Geometry: final body of the model. Coordinates: model frame, mm. Round coordinates to 2 decimals unless told otherwise and drop trailing zeros. Write each loop counter-clockwise with the first axis right and the second up, starting at its lowest first coordinate (ties: lowest second). Pieces come first, ordered by that corner, then holes. Notation, with made-up numbers: M 74,59 L 116,59 A25 ccw 116,75 Z; hole C 51,64 d10. An arc over 180 degrees is marked long. Answer as CSV lines item,"result". Start each with the question number.
Q1. Section query D-D on z = 0.75. Give the number of separate pieces and of enclosed holes in the cut face, and give its area (3 significant figures).
Q2. Section query C-C on x = 0. Output: boundary loops of the cut face in (y, z), and give its area (3 significant figures).
Q3. First-contact query: pin 1 (1 mm diameter, centred on x = -10, y = 5, fed in from -Z); pin 2 (0.8 mm diameter, centred on x = 8, z = 1, fed in from +Y); pin 3 (8 mm diameter, centred on x = 0, y = 9.144, fed in from -Z); pin 4 (0.5 mm diameter, centred on y = -3, z = 0.5, fed in from -X). Flat tips, straight axial feed; report the tip coordinate or a pass-through.
Q4. Ray query, probe 1 along Y at (x, z) = (-9, 1.45); probe 2 along X at (y, z) = (8, 1.55) (3 decimals); probe 3 along X at (y, z) = (7.25, 1.5) (3 decimals). Return the intervals inside material, ascending.
Q5. Section query B-B on y = 2.75. Output: boundary loops of the cut face in (x, z) (1 decimal), and give its area (3 significant figures).
Q6. Section query A-A on x = -5.08. Output: boundary loops of the cut face in (y, z), and give its area (3 significant figures).
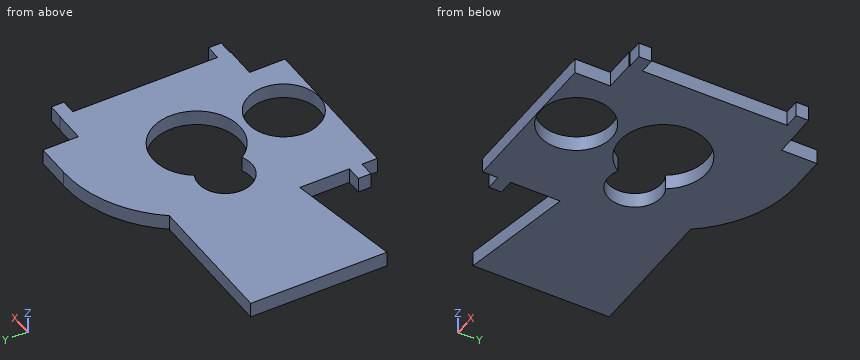
```python
from build123d import *

# Parameters (mm, degrees)
SKETCH1_R           = 3.7592
SKETCH1_W           = 1.5875
SKETCH1_H           = 1.3208
BOSS_EXTRUDE1_DEPTH = 1.5875
CUT_EXTRUDE1_REACH  = 32.926


with BuildPart() as part:
    # Sketch1 → Boss-Extrude1 (new body)
    # profile 1 of 6: a face of its own
    with BuildSketch(Plane.XY):
        with BuildLine():
            Line((2.54, 21.59), (9.525, 21.59))
            Line((9.525, 21.59), (9.525, -3.81))
            Line((9.525, -3.81), (-10.16, -3.81))
            Line((-10.16, -3.81), (-10.16, 8.89))
            ThreePointArc((-10.16, 8.89), (-6.440256121, 17.870256121), (2.54, 21.59))
        make_face()
        Circle(SKETCH1_R, mode=Mode.SUBTRACT)
        with BuildLine():
            ThreePointArc((-3.82905, 11.642311449), (-7.874, 9.144), (-3.82905, 6.645688551))
            ThreePointArc((-3.82905, 6.645688551), (4.572, 9.144), (-3.82905, 11.642311449))
        make_face(mode=Mode.SUBTRACT)
    # profile 2 of 6: a face of its own
    with BuildSketch(Plane.XY):
        with Locations((-10.95375, -1.5494)):
            Rectangle(SKETCH1_W, SKETCH1_H)
    # profile 3 of 6: a face of its own
    with BuildSketch(Plane.XY):
        with Locations((10.31875, 17.1704)):
            Rectangle(SKETCH1_W, SKETCH1_H)
    # profile 4 of 6: a face of its own
    with BuildSketch(Plane.XY):
        with Locations((10.31875, 0.6604)):
            Rectangle(SKETCH1_W, SKETCH1_H)
    # profile 5 of 6: a face of its own
    with BuildSketch(Plane.XY):
        with BuildLine():
            ThreePointArc((-10.16, 8.89), (-9.508277885, 12.906092628), (-7.62, 16.51))
            Line((-7.62, 16.51), (-22.084921519, 16.51))
            Line((-22.084921519, 16.51), (-22.084921519, 2.212007412))
            Line((-22.084921519, 2.212007412), (-10.16, 4.318))
            Line((-10.16, 4.318), (-10.16, 8.89))
        make_face()
    # profile 6 of 6: a face of its own
    with BuildSketch(Plane.XY):
        with BuildLine():
            ThreePointArc((-10.16, 8.89), (-9.508277885, 12.906092628), (-7.62, 16.51))
            Line((-7.62, 16.51), (-22.084921519, 16.51))
            Line((-22.084921519, 16.51), (-22.084921519, 2.212007412))
            Line((-22.084921519, 2.212007412), (-10.16, 4.318))
            Line((-10.16, 4.318), (-10.16, 8.89))
        make_face()
    extrude(amount=BOSS_EXTRUDE1_DEPTH)

    # Sketch2 → Cut-Extrude1 (cut, up to next)
    with BuildSketch(Plane.XY.offset(1.5875), mode=Mode.PRIVATE) as cut_extrude1_sk1:
        Polygon((6.223, -0.0889), (6.223, -3.81), (9.525, -3.81), (9.525, -3.0226), (9.525, -0.9144), (9.525, -0.0889), align=None)
    cut_extrude1_tool1 = extrude(cut_extrude1_sk1.sketch, amount=-CUT_EXTRUDE1_REACH, mode=Mode.PRIVATE) & part.part
    # Sketch2 → Cut-Extrude1 (cut, up to next)
    with BuildSketch(Plane.XY.offset(1.5875), mode=Mode.PRIVATE) as cut_extrude1_sk2:
        Polygon((9.525, 18.6944), (9.525, 20.8026), (9.525, 21.59), (6.223, 21.59), (6.223, 17.8689), (9.525, 17.8689), align=None)
    cut_extrude1_tool2 = extrude(cut_extrude1_sk2.sketch, amount=-CUT_EXTRUDE1_REACH, mode=Mode.PRIVATE) & part.part
    add(cut_extrude1_tool1.solids().sort_by_distance((7.874, -1.94945, 1.5875))[0], mode=Mode.SUBTRACT)
    add(cut_extrude1_tool2.solids().sort_by_distance((7.874, 19.72945, 1.5875))[0], mode=Mode.SUBTRACT)


solid = part.part
```
Entries:
1,separate pieces,"1"
1,enclosed holes,"2"
1,area,"485 mm^2"
2,outline,"M -3.81,0 L -3.76,0 L -3.76,1.59 L -3.81,1.59 Z; M 3.76,0 L 4.57,0 L 4.57,1.59 L 3.76,1.59 Z; M 13.72,0 L 21.33,0 L 21.33,1.59 L 13.72,1.59 Z"
2,area,"13.5 mm^2"
3,pin 1,"stops at z = 0"
3,pin 2,"stops at y = 17.87"
3,pin 3,"passes through"
3,pin 4,"stops at x = -10.16"
4,probe 1,"y = -3.81 to 16.51"
4,probe 2,"x = -22.085 to -7.629, 4.427 to 9.525"
4,probe 3,"x = -22.085 to -7.134, 4.161 to 9.525"
5,outline,"M -22.1,0 L -19,0 L -19,1.6 L -22.1,1.6 Z; M -10.2,0 L -2.6,0 L -2.6,1.6 L -10.2,1.6 Z; M 2.6,0 L 9.5,0 L 9.5,1.6 L 2.6,1.6 Z"
5,area,"27.9 mm^2"
6,outline,"M -3.81,0 L 6.35,0 L 6.35,1.59 L -3.81,1.59 Z; M 11.94,0 L 19.05,0 L 19.05,1.59 L 11.94,1.59 Z"
6,area,"27.4 mm^2"
